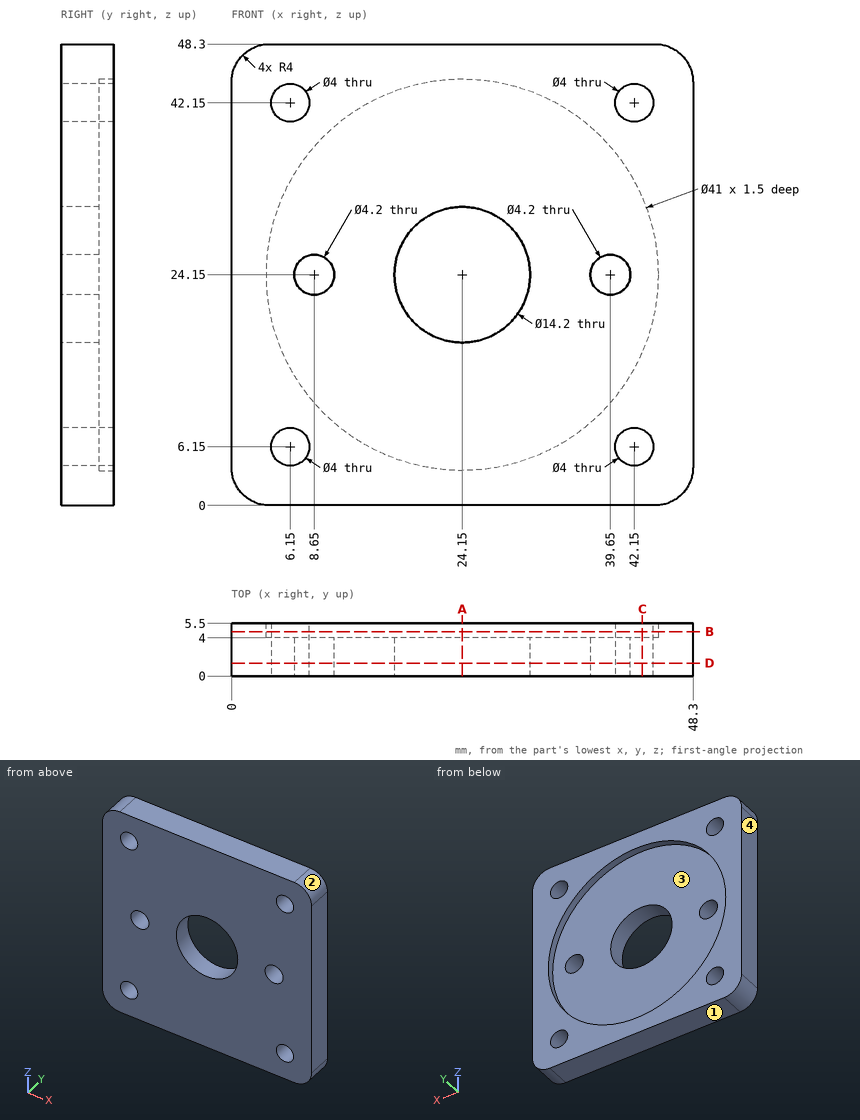
Verification items for this drawing (mm, ordinates from the low corner). Coordinates: 2 decimals unless noted, no trailing zeros. Loops run counter-clockwise (first coordinate to the right, second up) from the corner with the lowest first, then second, coordinate; pieces in that order, holes last. Notation, with made-up numbers: (44, 71.25) - (96, 71.25) arc R20 ccw to (96, 82.25) - close; hole circle Ø4 at (11, -13.5). An arc over 180 degrees is marked (long way). One line per item, written item: value. Start each with the question number.
(1) Cross-section at A-A on x = 24.15. Enter the section's corners in (y, z).
(2) Depth check by flat-ended pin: P1, Ø3, axis at x = 25, z = 16, coming from the +Y side. Enter the tip coordinate at first touch or a pass-through.
(3) Cross-section at C-C on x = 43. Enter the section's corners in (y, z), plus the area to 3 significant figures.
(4) Mould release check, pull along Z, two halves, no side actions. Record for the marked faces 1, 2, 3 and 4: released by +Z, released by -Z, zero draft, split by the parting line, or undercut.
(5) Material ranges on line 1 (X direction, y = 3.4, z = 6.15); line 2 (X direction, y = 1.3, z = 24.15), recorded low to high. Write a range as [from, to].
(6) Cross-section at D-D on y = 1.35. Enter the section's corners in (x, z), plus the area to 3 significant figures.
(7) Cross-section at B-B on y = 4.65. Enter the section's corners in (x, z), plus the area to 3 significant figures.
Results below:
1. outline: (0, 0) - (5.5, 0) - (5.5, 3.65) - (4, 3.65) - (4, 17.05) - (0, 17.05) - close; (0, 31.25) - (4, 31.25) - (4, 44.65) - (5.5, 44.65) - (5.5, 48.3) - (0, 48.3) - close
2. P1: stops at y = 4
3. outline: (0, 0) - (5.5, 0) - (5.5, 4.34) - (0, 4.34) - close; (0, 7.96) - (5.5, 7.96) - (5.5, 16.09) - (4, 16.09) - (4, 32.21) - (5.5, 32.21) - (5.5, 40.34) - (0, 40.34) - close; (0, 43.96) - (5.5, 43.96) - (5.5, 48.3) - (0, 48.3) - close
3. area: 202 mm2
4. face 1: released by -Z
4. face 2: released by +Z
4. face 3: undercut
4. face 4: zero draft
5. line 1: x = [0, 4.15], [8.15, 40.15], [44.15, 48.3]
5. line 2: x = [0, 6.55], [10.75, 17.05], [31.25, 37.55], [41.75, 48.3]
6. outline: (0, 4) arc R4 ccw to (4, 0) - (44.3, 0) arc R4 ccw to (48.3, 4) - (48.3, 44.3) arc R4 ccw to (44.3, 48.3) - (4, 48.3) arc R4 ccw to (0, 44.3) - close; hole circle Ø4 at (6.15, 6.15); hole circle Ø4 at (6.15, 42.15); hole circle Ø4.2 at (8.65, 24.15); hole circle Ø14.2 at (24.15, 24.15); hole circle Ø4.2 at (39.65, 24.15); hole circle Ø4 at (42.15, 6.15); hole circle Ø4 at (42.15, 42.15)
6. area: 2,080 mm2
7. outline: (0, 4) arc R4 ccw to (4, 0) - (44.3, 0) arc R4 ccw to (48.3, 4) - (48.3, 44.3) arc R4 ccw to (44.3, 48.3) - (4, 48.3) arc R4 ccw to (0, 44.3) - close; hole circle Ø41 at (24.15, 24.15); hole circle Ø4 at (6.15, 6.15); hole circle Ø4 at (6.15, 42.15); hole circle Ø4 at (42.15, 6.15); hole circle Ø4 at (42.15, 42.15)
7. area: 949 mm2
